```python
from build123d import *

# Parameters (mm, degrees)
F2_T = -1
F3_R = 1


with BuildPart() as f4:
    # F0 (on Front) → F4 (revolve)
    with BuildSketch(Plane.XZ):
        Polygon((0, 5.5), (0, 0), (55, 0), (55, 3), (38.5, 8), (36.5, 8), (36.5, 6.5), (11.5, 6.5), (11.5, 6), (3.5, 6), (3, 5.5), align=None)
    revolve(axis=Axis((5.4076574743, 0, 0), (1, 0, 0)))

    # F2
    f2_openings = [f4.faces().sort_by_distance(p)[0] for p in [
        (0, 0, 0),
        (55, 0, 0),
    ]]
    offset(amount=F2_T, openings=f2_openings, kind=Kind.INTERSECTION)

    # F3
    f3_edges = [f4.edges().sort_by_distance(p)[0] for p in [
        (55, 0, -3),
    ]]
    fillet(f3_edges, radius=F3_R)


solid = f4.part
```
For this review, take the finished solid that the model builds, in its own axes (mm). A direction names the side the tool comes from. Round coordinates to 2 decimals unless told otherwise and drop trailing zeros. Order: outer loops, then holes, each group sorted by start corner. A loop starts at its lowest first (then second) coordinate and runs counter-clockwise, first axis right, second up.
Q1. We need section B-B, the plane x = 39. Give the boundary of the cut face in (y, z).
Findings below:
outline: circle Ø15.7 at (0, 0); hole circle Ø13.61 at (0, 0)
Q2. We need section A-A, the plane x = 16.5. Give the boundary of the cut face in (y, z), plus the area to 3 significant figures.
Findings below:
outline: circle Ø13 at (0, 0); hole circle Ø11 at (0, 0)
area: 37.7 mm2
Q3. Machinability: for faces 4 (the conical face through (48.039, -1.535, 4.873)), 5 (the cylindrical face through (1.48, 5.37, -1.19)), 6 (the cylindrical face through (37.92, 2.681, 6.466)), which of the approach directions +Z, -Z, +X, -X, +Y, -Y give a long, thin tool a straight path to every point of the face, cutting with its end or side? Answer none if there is none.
Findings below:
face 4: +X
face 5: -X
face 6: none
Q4. Insertion check: P1, Ø6, axis at x = 9.5, y = -1, coming from the -Z side; P2, Ø1.5, axis at x = 41.5, z = 6.5, coming from the -Y side. Each pin has a flat end and moves straight along its axis. Give the tip position at first contact, or say it passes through.
Findings below:
P1: stops at z = -6.5
P2: stops at y = -4.22
Q5. Mouldability with a two-part tool opening along Y and no side actions: class faces 1 (the cylindrical face through (7, 0, -6)), 2 (the flat face through (11.5, 6, 2)), 3 (the flat face through (37.5, 4, -4)) as pulls with the +Y half, pulls with the -Y half, needs draft (parallel to the pull), parting line crosses it, or undercut.
Findings below:
face 1: parting line crosses it
face 2: needs draft
face 3: undercut
Q6. Wall thickness on line 1 (Z direction, x = 37.9, y = 0); line 2 (Y direction, x = 28, z = 0): over which ranges is each line inside the solid? List them lowest first.
Findings below:
line 1: z = -8 to -7, 7 to 8
line 2: y = -6.5 to -5.5, 5.5 to 6.5
